from build123d import *

# Parameters (mm, degrees)
SKETCH1_W           = 127
SKETCH1_H           = 76.2
BOSS_EXTRUDE1_DEPTH = 20.32
CUT_EXTRUDE2_DEPTH  = 150.493619931
SKETCH4_R           = 24.515114189
BOSS_EXTRUDE2_DEPTH = 25.4
SKETCH5_R           = 11.931407315
CUT_EXTRUDE3_DEPTH  = 156.002446432
SKETCH6_R           = 18.430592643
CUT_EXTRUDE4_DEPTH  = 7.62


with BuildPart() as part:
    # Sketch1 → Boss-Extrude1 (new body)
    with BuildSketch(Plane(origin=(0, 0, 0), x_dir=(1, 0, 0), z_dir=(0, 1, 0))):
        with Locations((63.5, 38.1)):
            Rectangle(SKETCH1_W, SKETCH1_H)
    extrude(amount=BOSS_EXTRUDE1_DEPTH)

    # Sketch2 → Cut-Extrude2 (cut, through all)
    with BuildSketch(Plane(origin=(0, 20.32, 0), x_dir=(1, 0, 0), z_dir=(0, 1, 0))):
        with BuildLine():
            Line((98.708096341, 20.973581043), (98.708096341, 54.953487977))
            ThreePointArc((98.708096341, 54.953487977), (106.486629254, 62.73202089), (114.265162167, 54.953487977))
            Line((114.265162167, 54.953487977), (114.265162167, 20.973581043))
            ThreePointArc((114.265162167, 20.973581043), (106.486629254, 13.195048131), (98.708096341, 20.973581043))
        make_face()
    extrude(amount=-CUT_EXTRUDE2_DEPTH, mode=Mode.SUBTRACT)

    # Sketch4 → Boss-Extrude2 (add)
    with BuildSketch(Plane(origin=(0, 20.32, 0), x_dir=(1, 0, 0), z_dir=(0, 1, 0))):
        with Locations(Location((31.75, 38.1, 0), (0, 0, 90))):
            Circle(SKETCH4_R)
    extrude(amount=BOSS_EXTRUDE2_DEPTH)

    # Sketch5 → Cut-Extrude3 (cut, through all)
    with BuildSketch(Plane(origin=(0, 45.72, 0), x_dir=(1, 0, 0), z_dir=(0, 1, 0))):
        with Locations(Location((31.75, 38.1, 0), (0, 0, 270))):
            Circle(SKETCH5_R)
    extrude(amount=-CUT_EXTRUDE3_DEPTH, mode=Mode.SUBTRACT)

    # Sketch6 → Cut-Extrude4 (cut)
    with BuildSketch(Plane(origin=(0, 45.72, 0), x_dir=(1, 0, 0), z_dir=(0, 1, 0))):
        with Locations(Location((31.75, 38.1, 0), (0, 0, 270))):
            Circle(SKETCH6_R)
    extrude(amount=-CUT_EXTRUDE4_DEPTH, mode=Mode.SUBTRACT)


solid = part.part
CAD build for the part. Positions are in the model's coordinates, mm. A direction names the side the tool comes from. Give positions to 0.01 mm unless a question says otherwise; leave off trailing zeros. Order: outer loops, then holes, each group sorted by start corner. A loop starts at its lowest first (then second) coordinate and runs counter-clockwise, first axis right, second up. Notation, with made-up numbers: (26, 52.25) - (52, 52.25) arc R12 cw to (52, 74.25) - close; hole circle Ø1 at (-18, 46.5). An arc over 180 degrees is marked (long way). Answer in a Markdown table with one row per item.
1. Saw through at D-D, the plane x = 86. Give the cut face in (y, z).
Data:
| item | result |
|---|---|
| outline | (0, -76.2) - (20.32, -76.2) - (20.32, 0) - (0, 0) - close |
2. Pull direction Z, two halves, no side cores. Call faces 1 (the cylindrical face through (41.811, 19.317, -31.686)), 2 (the cylindrical face through (106.32, 10.3, -62.73)), 3 (the flat face through (13, 45.72, -42)), 4 (the flat face through (63, 10, -76.2)): pulls with the +Z half, pulls with the -Z half, needs draft (parallel to the pull), parting line crosses it, or undercut.
Data:
| item | result |
|---|---|
| face 1 | undercut |
| face 2 | undercut |
| face 3 | needs draft |
| face 4 | pulls with the -Z half |
3. Saw through at A-A, the plane x = 31.75. Give the cut face in (y, z).
Data:
| item | result |
|---|---|
| outline | (0, -76.2) - (20.32, -76.2) - (20.32, -62.62) - (45.72, -62.62) - (45.72, -56.53) - (38.1, -56.53) - (38.1, -50.03) - (0, -50.03) - close; (0, -26.17) - (38.1, -26.17) - (38.1, -19.67) - (45.72, -19.67) - (45.72, -13.58) - (20.32, -13.58) - (20.32, 0) - (0, 0) - close |
4. Saw through at C-C, the plane y = 28.5. Give the cut face in (x, z), plus the area to 3 significant figures.
Data:
| item | result |
|---|---|
| outline | circle Ø49.03 at (31.75, -38.1); hole circle Ø23.86 at (31.75, -38.1) |
| area | 1,440 mm² |
5. Flat gauge pins, fed straight in: pin 1 (22 mm diameter, centred on x = 31.75, z = -38.1, fed in from +Y); pin 2 (8 mm diameter, centred on x = 13.5, y = 35, fed in from -Z); pin 3 (1.5 mm diameter, centred on x = 86.5, z = -32.5, fed in from +Y); pin 4 (8 mm diameter, centred on y = 36, z = -28, fed in from +X). Where does each tip first touch, or does it go through?
Data:
| item | result |
|---|---|
| pin 1 | passes through |
| pin 2 | stops at z = -58.05 |
| pin 3 | stops at y = 20.32 |
| pin 4 | stops at x = 55.49 |
6. Saw through at B-B, the plane z = -38.1. Give the cut face in (x, y), plus the area to 3 significant figures.
Data:
| item | result |
|---|---|
| outline | (0, 0) - (19.82, 0) - (19.82, 38.1) - (13.32, 38.1) - (13.32, 45.72) - (7.23, 45.72) - (7.23, 20.32) - (0, 20.32) - close; (43.68, 0) - (98.71, 0) - (98.71, 20.32) - (56.27, 20.32) - (56.27, 45.72) - (50.18, 45.72) - (50.18, 38.1) - (43.68, 38.1) - close; (114.27, 0) - (127, 0) - (127, 20.32) - (114.27, 20.32) - close |
| area | 2,320 mm² |
7. Tool access for faces 5 (the flat face through (32, 38.1, -26)), 6 (the flat face through (63, 0, -39)), 7 (the cylindrical face through (106.658, 10.302, -13.197)): list every direction of +Z, -Z, +X, -X, +Y, -Y with a clear straight run to the whole face (end or side of a thin tool).
Data:
| item | result |
|---|---|
| face 5 | +Y |
| face 6 | +Z, -Z, +X, -X, -Y |
| face 7 | +Y, -Y |
8. Probe probe 1 along Z at (x, y) = (31, 27); probe 2 along Z at (x, y) = (31, 12); probe 3 along X at (y, z) = (28, -38.1). List the from-to ranges inside material, lowest first. Write a range as [from, to].
Data:
| item | result |
|---|---|
| probe 1 | z = [-62.6, -50.01], [-26.19, -13.6] |
| probe 2 | z = [-76.2, -50.01], [-26.19, 0] |
| probe 3 | x = [7.23, 19.82], [43.68, 56.27] |
